Here's how the part is built. I have some questions about the finished solid (model axes, mm). Face numbers are marked on the shaded views. Give positions to 0.01 mm unless a question says otherwise; leave off trailing zeros. Order: outer loops, then holes, each group sorted by start corner. A loop starts at its lowest first (then second) coordinate and runs counter-clockwise, first axis right, second up. Notation, with made-up numbers: M 46.5,-11 L 105.5,-11 A15 cw 105.5,15 Z; hole C 62,55.5 d9. An arc over 180 degrees is marked long. Use one line per item in the form item = value.
from build123d import *

# Parameters (mm, degrees)
F0_R     = 3.175
F0_R_2   = 1.5875
F1_DEPTH = 2.54
F2_DEPTH = 25.4
F3_R     = 12.69999
F4_DEPTH = 31.75


# Not quite as in the source:
# - a fillet or chamfer is up to 0.001 mm smaller than in the source, because OpenCascade refuses the exact size


with BuildPart() as f1:
    # F0 (on Top) → F1 (new body)
    with BuildSketch(Plane.XY):
        Polygon((12.7, 144.78), (0, 144.78), (-12.7, 144.78), (-12.7, -12.7), (0, -12.7), (12.7, -12.7), align=None)
        Circle(F0_R, mode=Mode.SUBTRACT)
        with Locations((0, 132.08)):
            Circle(F0_R, mode=Mode.SUBTRACT)
        with Locations((0, 132.08)):
            Circle(F0_R)
        with Locations((0, 132.08)):
            Circle(F0_R_2, mode=Mode.SUBTRACT)
        with Locations((0, 132.08)):
            Circle(F0_R_2)
        Circle(F0_R)
        Circle(F0_R_2, mode=Mode.SUBTRACT)
        Circle(F0_R_2)
    extrude(amount=-F1_DEPTH)

    # F0 (on Top) → F2 (join)
    with BuildSketch(Plane.XY):
        with Locations((0, 132.08)):
            Circle(F0_R)
        with Locations((0, 132.08)):
            Circle(F0_R_2, mode=Mode.SUBTRACT)
        Circle(F0_R)
        Circle(F0_R_2, mode=Mode.SUBTRACT)
        with Locations((0, 132.08)):
            Circle(F0_R_2)
        Circle(F0_R_2)
    extrude(amount=F2_DEPTH)

    # F3 (radius 12.7 in the source; OpenCascade refuses exactly that, so slightly less here)
    f3_edges = [f1.edges().sort_by_distance(p)[0] for p in [
        (12.7, 144.78, -1.27),
        (-12.7, 144.78, -1.27),
        (-12.7, -12.7, -1.27),
        (12.7, -12.7, -1.27),
    ]]
    fillet(f3_edges, radius=F3_R)

    # F0 (on Top) → F4 (join)
    with BuildSketch(Plane.XY):
        Circle(F0_R_2)
        with Locations((0, 132.08)):
            Circle(F0_R_2)
    extrude(amount=F4_DEPTH)


solid = f1.part
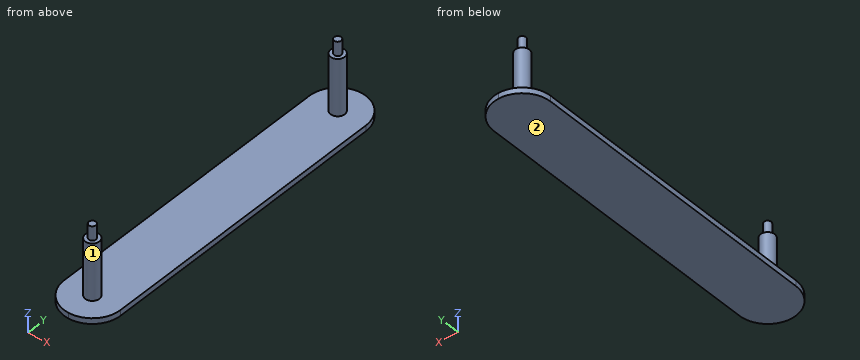
Q1. I want a section at B-B on z = 29.5. Write out the boundary of the cut face in (x, y) (1 decimal), then the cut area to 3 significant figures.
Found:
outline = C 0,0 d3.2; C 0,132.1 d3.2
area = 15.8 mm²
Q2. I want a section at A-A on z = 9.5. Write out the boundary of the cut face in (x, y) (3 decimals).
Found:
outline = C 0,0 d6.35; C 0,132.08 d6.35
Q3. I need wall thicknesses on L1, parallel to Y at x = 0.25, z = 5; L2, parallel to Z at x = -8, y = 103.5; L3, parallel to Y at x = -0.5, z = 18.5. Which ranges of each line are inside material? Lowest first, please.
Found:
L1 = -3.17 to 3.17, 128.91 to 135.25
L2 = -2.54 to 0
L3 = -3.14 to 3.14, 128.94 to 135.22
Q4. I want a section at D-D on x = 10. Write out the boundary of the cut face in (y, z).
Found:
outline = M -7.83,-2.54 L 139.91,-2.54 L 139.91,0 L -7.83,0 Z
Q5. I'm going to push flat-ended pins straight in: pin 1 Ø1 at (x, y) = (1.5, 22) entering from +Z; pin 2 Ø1 at (x, z) = (-2.5, 19.5) entering from +Y; pin 3 Ø5 at (y, z) = (5, 15.5) entering from +X. Where does each tip first touch, or does it pass through?
Found:
pin_1 = 0
pin_2 = 134.55
pin_3 = 1.96
Q6. I want a section at C-C on y = 84.5. Write out the boundary of the cut face in (x, z).
Found:
outline = M -12.7,-2.54 L 12.7,-2.54 L 12.7,0 L -12.7,0 Z
Q7. Thinking about a two-plate mould opening in Y: for the marked faces 1 and 2, which applies, +Y half, -Y half, draft (parallel to the pull), parting line (faces both ways), or undercut?
Found:
face_1 = undercut
face_2 = draft
